```python
from build123d import *

# Parameters (mm, degrees)
SKETCH1_W           = 99.06
SKETCH1_H           = 71.12
BOSS_EXTRUDE1_DEPTH = 40
FILLET1_R           = 5.08
CUT_EXTRUDE2_DEPTH  = 35


with BuildPart() as part:
    # Sketch1 → Boss-Extrude1 (new body)
    with BuildSketch(Plane.XY):
        with Locations((0.589485294, -0.109632353)):
            Rectangle(SKETCH1_W, SKETCH1_H)
    extrude(amount=BOSS_EXTRUDE1_DEPTH)

    # Fillet1
    fillet1_edges = [part.edges().sort_by_distance(p)[0] for p in [
        (-48.940514706, 35.450367647, 20),
        (50.119485294, 35.450367647, 20),
        (50.119485294, -35.669632353, 20),
        (-48.940514706, -35.669632353, 20),
    ]]
    fillet(fillet1_edges, radius=FILLET1_R)

    # Sketch2 → Cut-Extrude2 (cut)
    with BuildSketch(Plane.XY.offset(40)):
        with BuildLine():
            Line((47.579485294, -30.589632353), (47.579485294, 30.370367647))
            ThreePointArc((47.579485294, 30.370367647), (46.835536518, 32.166418871), (45.039485294, 32.910367647))
            Line((45.039485294, 32.910367647), (-43.860514706, 32.910367647))
            ThreePointArc((-43.860514706, 32.910367647), (-45.65656593, 32.166418871), (-46.400514706, 30.370367647))
            Line((-46.400514706, 30.370367647), (-46.400514706, -30.589632353))
            ThreePointArc((-46.400514706, -30.589632353), (-45.65656593, -32.385683577), (-43.860514706, -33.129632353))
            Line((-43.860514706, -33.129632353), (45.039485294, -33.129632353))
            ThreePointArc((45.039485294, -33.129632353), (46.835536518, -32.385683577), (47.579485294, -30.589632353))
        make_face()
    extrude(amount=-CUT_EXTRUDE2_DEPTH, mode=Mode.SUBTRACT)


solid = part.part
```
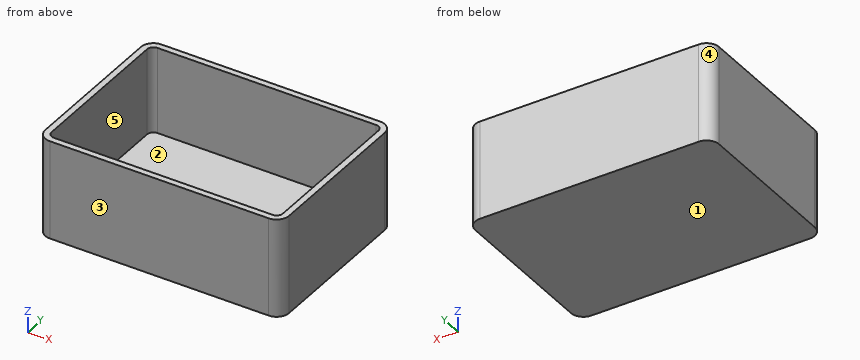
CAD build for the part. Positions are in the model's coordinates, mm. Face numbers are marked on the shaded views. A direction names the side the tool comes from. Coordinates: 2 decimals unless noted, no trailing zeros. Write each loop counter-clockwise with the first axis right and the second up, starting at its lowest first coordinate (ties: lowest second). Pieces come first, ordered by that corner, then holes.
(1) 3-axis set-ups, long thin cutter, end or side, ignore diameter. For the marked faces 1 and 2: which of +Z, -Z, +X, -X, +Y, -Y reach the whole face in a straight line?
(2) Cut at A-A, the plane y = 18. List the corners of the cut face in (x, z).
(3) Two-plate mould, pull along Y, no slides. Class the marked faces 3, 4 and 5: +Y half, -Y half, draft (parallel to the pull), parting line (faces both ways), or undercut.
(4) Drill centre lines: probe 1 along Y at (x, z) = (40, 31); probe 2 along X at (y, z) = (29, 27); probe 3 along Z at (x, y) = (22.5, -32). Where is each one in solid material? Low to high.
(5) Flat gauge pin, fed straight in: pin 1 (2 mm diameter, centred on x = -30.5, y = -26, fed in from +Z). Where does the tip first touch, or does it go through?
(6) Cut at C-C, the plane x = 1. List the corners of the cut face in (y, z), and give its area (3 significant figures).
(7) Cut at B-B, the plane z = 13. List the corners of the cut face in (x, y), and give its area (3 significant figures).
Geometry says:
1. face 1: -Z, +X, -X, +Y, -Y
1. face 2: +Z
2. outline: (-48.94, 0) - (50.12, 0) - (50.12, 40) - (47.58, 40) - (47.58, 5) - (-46.4, 5) - (-46.4, 40) - (-48.94, 40) - close
3. face 3: -Y half
3. face 4: +Y half
3. face 5: undercut
4. probe 1: y = -35.67 to -33.13, 32.91 to 35.45
4. probe 2: x = -48.94 to -46.4, 47.58 to 50.12
4. probe 3: z = 0 to 5
5. pin 1: stops at z = 5
6. outline: (-35.67, 0) - (35.45, 0) - (35.45, 40) - (32.91, 40) - (32.91, 5) - (-33.13, 5) - (-33.13, 40) - (-35.67, 40) - close
6. area: 533 mm2
7. outline: (-48.94, -30.59) arc R5.08 ccw to (-43.86, -35.67) - (45.04, -35.67) arc R5.08 ccw to (50.12, -30.59) - (50.12, 30.37) arc R5.08 ccw to (45.04, 35.45) - (-43.86, 35.45) arc R5.08 ccw to (-48.94, 30.37) - close; hole (-46.4, -30.59) arc R2.54 ccw to (-43.86, -33.13) - (45.04, -33.13) arc R2.54 ccw to (47.58, -30.59) - (47.58, 30.37) arc R2.54 ccw to (45.04, 32.91) - (-43.86, 32.91) arc R2.54 ccw to (-46.4, 30.37) - close
7. area: 822 mm2
